Could you check a few things on this model? Use its own coordinates, in mm. Round coordinates to 2 decimals unless told otherwise and drop trailing zeros. Write each loop counter-clockwise with the first axis right and the second up, starting at its lowest first coordinate (ties: lowest second). Pieces come first, ordered by that corner, then holes. Notation, with made-up numbers: (31.5, 51) -> (50.5, 51) arc R22 cw to (50.5, 82) -> close; hole circle Ø4 at (68.5, -14). An arc over 180 degrees is marked (long way). One line per question, with ' | ' between items. Start each with the question number.
1. Imagine slicing it at A-A, the plane x = 3. List the corners of the cut face in (y, z) for me.
2. For pin 1 Ø3.5 at (y, z) = (0, 0) entering from -X; pin 2 Ø2 at (x, z) = (3.5, -0.5) entering from +Y; pin 3 Ø1.5 at (x, y) = (5.5, -1) entering from +Z; pin 4 Ø3 at (y, z) = (-1.5, 0) entering from +X, each with a flat end and sliding along its axis, tell me the tip position at first contact or that it passes through.
3. Imagine slicing it at B-B, the plane x = 4.25. List the corners of the cut face in (y, z) for me (3 decimals).
4. If I drill on line 1 along Y through (x, z) = (5.5, 6.25); line 2 along X through (y, z) = (-2, -2); line 3 along Z through (x, y) = (3, 0), over which ranges is the centre line in solid material (lowest first)? Write a range as [from, to].
5. Thinking about a two-plate mould opening in X: for faces 1 (the conical face through (5.229, -2.218, -7.045)), 2 (the flat face through (0, 2.4, 0.1)), 3 (the flat face through (6, 0, -3.5)), 4 (the cylindrical face through (2.03, -0.29, 2.23)), which applies, released by +X, released by -X, zero draft, split by the parting line, or undercut?
Autodesk Inventor part; units mm, degrees
ref_plane "Work Plane1" through (7, 0, 0) normal (1, 0, 0) x (0, 1, 0)
ref_plane "XZ Plane" through (0, 0, 0) normal (0, 1, 0) x (-1, 0, 0)
ref_plane "XY Plane" through (0, 0, 0) normal (0, 0, 1) x (1, 0, 0)
ref_plane "Work Plane1" through (7, 0, 0) normal (1, 0, 0) x (0, 1, 0)
sketch "Sketch1" plane through (0, 0, 0) normal (0, 1, 0) x (-1, 0, 0)
  line L0 (0, 0) -> (-10, 0)
  line L1 (0, 0) -> (0, -10)
  line L2 (-10, 0) -> (-10, -5)
  line L3 (-10, -5) -> (0, -10)
  dimension "d0" = 10
  dimension "d1" = 10
  dimension "d2" = 5
revolve "Revolution1" add sketch "Sketch1" angle 360 about axis through (0, 0, 0) along (1, 0, 0)
sketch "Sketch2" plane through (7, 0, 0) normal (1, 0, 0) x (0, 1, 0)
  circle A0 centre (0, 0) radius 2.25
  dimension "d5" = 4.5
extrude "Extrusion1" cut sketch "Sketch2" along normal blind 2 and the other way blind 10
sketch "Sketch3" plane through (7, 0, 0) normal (1, 0, 0) x (0, 1, 0)
  line L0 (-3.5, 3.5) -> (3.5, 3.5)
  line L1 (3.5, 3.5) -> (3.5, -3.5)
  line L2 (3.5, -3.5) -> (-3.5, -3.5)
  line L3 (-3.5, -3.5) -> (-3.5, 3.5)
  line L4 (-3.5, 3.5) -> (3.5, -3.5) construction
  line L5 (3.5, 3.5) -> (-3.5, -3.5) construction
  line L6 (-3.5, 3.5) -> (3.5, 3.5)
  line L7 (3.5, 3.5) -> (3.5, 13.5)
  line L8 (3.5, 13.5) -> (-3.5, 13.5)
  line L9 (-3.5, 13.5) -> (-3.5, 3.5)
  point P0 (0, 0)
  dimension "d18" = 7
  dimension "d19" = 7
  dimension "d20" = 7
  dimension "d21" = 10
extrude "Extrusion2" cut sketch "Sketch3" against normal blind 3
sketch "Sketch5" plane through (9, 0, 0) normal (-1, 0, 0) x (0, 0, 1)
  circle A0 centre (0, 0) radius 2.25
extrude "Extrusion3" add sketch "Sketch5" along normal up to surface (2 mm away)
sketch "Sketch7" plane through (10, 0, 0) normal (1, 0, 0) x (0, 0, -1)
  circle A0 centre (0, 0) radius 5
extrude "Extrusion4" [suppressed]
fillet "Fillet2" radius 8 1 edges at (10, 0, 5)
properties part number "stollen_m4_vierkant_rounded"
Geometry results:
1) outline: circle Ø17 at (0, 0); hole circle Ø4.5 at (0, 0)
2) pin 1: stops at x = 7 | pin 2: stops at y = 8.74 | pin 3: stops at z = -3.5 | pin 4: stops at x = 10
3) outline: (-3.5, -3.5) -> (-3.5, 7.054) arc R7.875 ccw (long way) to (3.5, 7.054) -> (3.5, -3.5) -> close
4) line 1: y = [-3.67, -3.5], [3.5, 3.67] | line 2: x = [0, 4], [7, 9.5] | line 3: z = [-8.5, -2.25], [2.25, 8.5]
5) face 1: released by +X | face 2: released by -X | face 3: undercut | face 4: zero draft
